For this review, take the finished solid that the model builds, in its own axes (mm). Face numbers are marked on the shaded views. A direction names the side the tool comes from. Coordinates: 2 decimals unless noted, no trailing zeros. Write each loop counter-clockwise with the first axis right and the second up, starting at its lowest first coordinate (ties: lowest second). Pieces come first, ordered by that corner, then holes.
1) For the marked faces 4 and 5, list the 3-axis set-ups (+Z, -Z, +X, -X, +Y, -Y) from which the entire face can be reached by the end or side of a thin tool; tool diameter is ignored.
2) Mouldability with a two-part tool opening along Y and no side actions: class the marked faces 1, 2 and 3 as pulls with the +Y half, pulls with the -Y half, needs draft (parallel to the pull), parting line crosses it, or undercut.
3) We need section A-A on z = 21.5. Write out the cut boundary in (x, y).
4) We need section C-C on x = -15.5. Write out the cut boundary in (y, z).
5) To check wall thickness, follow line 1 along Y through (x, z) = (50, -0.85); line 2 along Z through (x, y) = (-79, -39.5); line 3 along Y through (x, z) = (18.5, 5). State the ranges of each line that lie inside material, in increasing order.
6) Insertion check: P1, Ø5, axis at x = 1, z = 29, coming from the -Y side; P2, Ø1, axis at x = -48, z = 16.5, coming from the -Y side; P3, Ø1.5, axis at x = -76, y = -44, coming from the -Z side; P4, Ø4, axis at x = -100, y = -64.47, coming from the -Z side. Each pin has a flat end and moves straight along its axis. Give the tip position at first contact, or say it passes through.
7) We need section B-B on y = -38. Write out the cut boundary in (x, z).
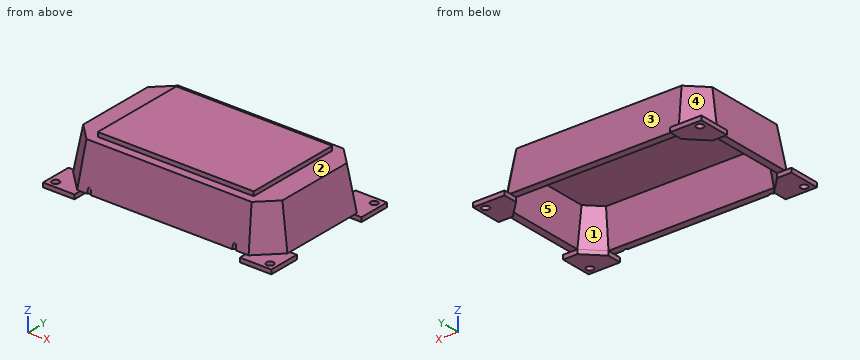
from build123d import *

# Parameters (mm, degrees)
BOSS_EXTRUDE1_DEPTH     = 30
BOSS_EXTRUDE1_TAPER     = 10
SHELL1_T                = -5
SKETCH4_R               = 1.5
CUT_EXTRUDE1_DEPTH      = 15
SKETCH5_W               = 109.114976024
SKETCH5_H               = 67.775815427
BOSS_EXTRUDE3_DEPTH     = 3
BOSS_EXTRUDE5_DEPTH     = 3
MIRROR5_COPY_1_DEPTH    = 3
CUT_EXTRUDE2_START      = -4
SKETCH9_R               = 2.5
CUT_EXTRUDE2_DEPTH      = 38
MIRROR7_START           = -4
MIRROR7_COPY_1_SKETCH_R = 2.5
MIRROR7_COPY_1_DEPTH    = 38


with BuildPart() as part:
    # Sketch1 → Boss-Extrude1 (new body)
    with BuildSketch(Plane.XY):
        Polygon((-100, 10.531931481), (-100, -49.468068519), (-85, -64.468068519), (35, -64.468068519), (50, -49.468068519), (50, 10.531931481), (35, 25.531931481), (-85, 25.531931481), align=None)
    extrude(amount=BOSS_EXTRUDE1_DEPTH, taper=BOSS_EXTRUDE1_TAPER)

    # Shell1
    shell1_openings = [part.faces().sort_by_distance(p)[0] for p in [
        (-25, -19.468068519, 0),
    ]]
    offset(amount=SHELL1_T, openings=shell1_openings, kind=Kind.INTERSECTION)

    # Sketch4 → Cut-Extrude1 (cut)
    with BuildSketch(Plane(origin=(0, 0, -7), x_dir=(-1, 0, 0), z_dir=(0, 0, -1))):
        with Locations((-24.758515909, -65.141240386)):
            Circle(SKETCH4_R)
    cut_extrude1 = extrude(amount=-CUT_EXTRUDE1_DEPTH, mode=Mode.SUBTRACT)

    # Mirror1: Cut-Extrude1 across plane
    add(cut_extrude1.mirror(Plane(origin=(-26.029584976, 0, 0), x_dir=(0, 0, 1), z_dir=(1, 0, 0))), mode=Mode.SUBTRACT)

    # Sketch5 → Boss-Extrude3 (add)
    with BuildSketch(Plane.XY.offset(30)):
        with Locations((-25, -19.468068519)):
            Rectangle(SKETCH5_W, SKETCH5_H)
    extrude(amount=BOSS_EXTRUDE3_DEPTH)

    # Sketch8 → Boss-Extrude5 (add)
    with BuildSketch(Plane(origin=(0, 0, 0), x_dir=(-1, 0, 0), z_dir=(0, 0, -1))):
        Polygon((-54.922866941, 8.42891411), (-44.922866941, 8.42891411), (-32.896982629, 20.454798422), (-32.896982629, 30.454798422), (-54.922866941, 30.454798422), align=None)
    boss_extrude5 = extrude(amount=BOSS_EXTRUDE5_DEPTH)

    # Mirror4: Boss-Extrude5 across plane
    add(boss_extrude5.mirror(Plane.ZY.offset(25)))

    # Mirror5: Boss-Extrude5 across plane
    add(boss_extrude5.mirror(Plane.ZX.offset(-19.468068519)))

    # Mirror5 copy 1 sketch → Mirror5 copy 1 (add)
    with BuildSketch(Plane(origin=(-50, -38.936137038, 0), x_dir=(1, 0, 0), z_dir=(0, 0, -1))):
        Polygon((-54.922866941, 8.42891411), (-44.922866941, 8.42891411), (-32.896982629, 20.454798422), (-32.896982629, 30.454798422), (-54.922866941, 30.454798422), align=None)
    extrude(amount=MIRROR5_COPY_1_DEPTH)

    # Sketch9 → Cut-Extrude2 (cut)
    with BuildSketch(Plane.XY.offset(CUT_EXTRUDE2_START)):
        with Locations((50, -64.468068519)):
            Circle(SKETCH9_R)
    cut_extrude2 = extrude(amount=CUT_EXTRUDE2_DEPTH, mode=Mode.SUBTRACT)

    # Mirror6: Cut-Extrude2 across plane
    add(cut_extrude2.mirror(Plane.ZY.offset(25)), mode=Mode.SUBTRACT)

    # Mirror7: Cut-Extrude2 across plane
    add(cut_extrude2.mirror(Plane.ZX.offset(-19.468068519)), mode=Mode.SUBTRACT)

    # Mirror7 copy 1 sketch → Mirror7 copy 1 (cut)
    with BuildSketch(Plane(origin=(-50, -38.936137038, 0), x_dir=(-1, 0, 0), z_dir=(0, 0, 1)).offset(MIRROR7_START)):
        with Locations((50, -64.468068519)):
            Circle(MIRROR7_COPY_1_SKETCH_R)
    extrude(amount=MIRROR7_COPY_1_DEPTH, mode=Mode.SUBTRACT)


solid = part.part
Result:
1. face 4: +Z, -X, +Y
1. face 5: -Z
2. face 1: undercut
2. face 2: needs draft
2. face 3: pulls with the +Y half
3. outline: (-96.21, -47.9) - (-83.43, -60.68) - (33.43, -60.68) - (46.21, -47.9) - (46.21, 8.96) - (33.43, 21.74) - (-83.43, 21.74) - (-96.21, 8.96) - close; hole (-91.13, -45.79) - (-81.33, -55.6) - (31.33, -55.6) - (41.13, -45.79) - (41.13, 6.86) - (31.33, 16.66) - (-81.33, 16.66) - (-91.13, 6.86) - close
4. outline: (-64.47, 0) - (-59.39, 0) - (-54.98, 25) - (16.05, 25) - (20.45, 0) - (25.53, 0) - (20.24, 30) - (14.42, 30) - (14.42, 33) - (-53.36, 33) - (-53.36, 30) - (-59.18, 30) - close
5. line 1: y = -69.39 to -66.97, -61.97 to -47.37, 8.43 to 23.03, 28.03 to 30.45
5. line 2: z = 25 to 33
5. line 3: y = -63.59 to -58.51, 19.57 to 24.65
6. P1: stops at y = -59.8
6. P2: stops at y = -61.65
6. P3: stops at z = 25
6. P4: passes through
7. outline: (-100, 0) - (-94.92, 0) - (-90.51, 25) - (40.51, 25) - (44.92, 0) - (50, 0) - (44.71, 30) - (29.56, 30) - (29.56, 33) - (-79.56, 33) - (-79.56, 30) - (-94.71, 30) - close
